Geometry: final body of the model. Coordinates: model frame, mm. A direction names the side the tool comes from. Give positions to 0.01 mm unless a question says otherwise; leave off trailing zeros. Order: outer loops, then holes, each group sorted by start corner. A loop starts at its lowest first (then second) coordinate and runs counter-clockwise, first axis right, second up. Notation, with made-up numbers: M -8,66.5 L 30,66.5 A32 ccw 30,101.5 Z; hole C -18.75,14.25 d9. An arc over 180 degrees is marked long. One line per item, written item: value. Start each with the question number.
```python
from build123d import *

# Parameters (mm, degrees)
F0_R     = 11
F1_DEPTH = 7


with BuildPart() as f1:
    # F0 (on Top) → F1 (new body)
    with BuildSketch(Plane.XY):
        with BuildLine():
            ThreePointArc((9.403824, 18.776797), (0, 21), (-9.403824, 18.776797))
            ThreePointArc((-9.403824, 18.776797), (-12.34349, 16.989357), (-14.951853, 14.745918))
            ThreePointArc((-14.951853, 14.745918), (-19.972187, 6.489357), (-20.763736, -3.141219))
            ThreePointArc((-20.763736, -3.141219), (-19.972187, -6.489357), (-18.644578, -9.663318))
            ThreePointArc((-18.644578, -9.663318), (-12.34349, -16.989357), (-3.42887, -20.718177))
            ThreePointArc((-3.42887, -20.718177), (0, -21), (3.42887, -20.718177))
            ThreePointArc((3.42887, -20.718177), (12.34349, -16.989357), (18.644578, -9.663318))
            ThreePointArc((18.644578, -9.663318), (19.972187, -6.489357), (20.763736, -3.141219))
            ThreePointArc((20.763736, -3.141219), (20.940851, -1.575046), (21, 0))
            ThreePointArc((21, 0), (19.429217, 7.969036), (14.951853, 14.745918))
            ThreePointArc((14.951853, 14.745918), (12.34349, 16.989357), (9.403824, 18.776797))
        make_face()
        Circle(F0_R, mode=Mode.SUBTRACT)
        with BuildLine():
            Line((-0.986697, 24.434563), (-0.986697, 39.987829))
            ThreePointArc((-0.986697, 39.987829), (-4.11855, 39.787404), (-7.225052, 39.342072))
            Line((-7.225052, 39.342072), (-9.403824, 18.776797))
            ThreePointArc((-9.403824, 18.776797), (0, 21), (9.403824, 18.776797))
            Line((9.403824, 18.776797), (7.225052, 39.342072))
            ThreePointArc((7.225052, 39.342072), (4.11855, 39.787404), (0.986697, 39.987829))
            Line((0.986697, 39.987829), (0.986697, 24.434563))
            Line((0.986697, 24.434563), (-0.986697, 24.434563))
        make_face()
        with BuildLine():
            Line((35.18387, 19.028802), (14.951853, 14.745918))
            ThreePointArc((14.951853, 14.745918), (19.429217, 7.969036), (21, 0))
            ThreePointArc((21, 0), (20.940851, -1.575046), (20.763736, -3.141219))
            Line((20.763736, -3.141219), (39.649198, 5.285936))
            ThreePointArc((39.649198, 5.285936), (39.112772, 8.37801), (38.335591, 11.418514))
            Line((38.335591, 11.418514), (23.543556, 6.612291))
            Line((23.543556, 6.612291), (22.933744, 8.4891))
            Line((22.933744, 8.4891), (37.725779, 13.295323))
            ThreePointArc((37.725779, 13.295323), (36.567368, 16.211958), (35.18387, 19.028802))
        make_face()
        with BuildLine():
            Line((28.96988, -27.581626), (18.644578, -9.663318))
            ThreePointArc((18.644578, -9.663318), (12.34349, -16.989357), (3.42887, -20.718177))
            Line((3.42887, -20.718177), (17.2795, -36.075184))
            ThreePointArc((17.2795, -36.075184), (20.054472, -34.609509), (22.706001, -32.930799))
            Line((22.706001, -32.930799), (13.564021, -20.347942))
            Line((13.564021, -20.347942), (15.16053, -19.188011))
            Line((15.16053, -19.188011), (24.30251, -31.770867))
            ThreePointArc((24.30251, -31.770867), (26.718427, -29.767863), (28.96988, -27.581626))
        make_face()
        with BuildLine():
            ThreePointArc((-3.42887, -20.718177), (-12.34349, -16.989357), (-18.644578, -9.663318))
            Line((-18.644578, -9.663318), (-28.96988, -27.581626))
            ThreePointArc((-28.96988, -27.581626), (-26.718427, -29.767863), (-24.30251, -31.770867))
            Line((-24.30251, -31.770867), (-15.16053, -19.188011))
            Line((-15.16053, -19.188011), (-13.564021, -20.347942))
            Line((-13.564021, -20.347942), (-22.706001, -32.930799))
            ThreePointArc((-22.706001, -32.930799), (-20.054472, -34.609509), (-17.2795, -36.075184))
            Line((-17.2795, -36.075184), (-3.42887, -20.718177))
        make_face()
        with BuildLine():
            ThreePointArc((-20.763736, -3.141219), (-19.972187, 6.489357), (-14.951853, 14.745918))
            Line((-14.951853, 14.745918), (-35.18387, 19.028802))
            ThreePointArc((-35.18387, 19.028802), (-36.567368, 16.211958), (-37.725779, 13.295323))
            Line((-37.725779, 13.295323), (-22.933744, 8.4891))
            Line((-22.933744, 8.4891), (-23.543556, 6.612291))
            Line((-23.543556, 6.612291), (-38.335591, 11.418514))
            ThreePointArc((-38.335591, 11.418514), (-39.112772, 8.37801), (-39.649198, 5.285936))
            Line((-39.649198, 5.285936), (-20.763736, -3.141219))
        make_face()
    extrude(amount=F1_DEPTH)


solid = f1.part
```
Q1. Section query B-B on y = 0. Return loops of the section in (x, z), and give its area (3 significant figures).
Q2. Mould query, pull axis Y, two halves, no side actions, for faces 1 (the face through (6, 11, 0)), 2 (the face through (-30.34, 1.13, 3.45)), 3 (the face through (-4.075, 39.792, 3.451)). Classes: +Y half, -Y half, draft (parallel to the pull), parting line (faces both ways), or undercut.
Q3. Section query C-C on x = 26.5. Return loops of the section in (y, z), and give its area (3 significant figures).
Q4. Contact query for flat-ended pins moving along their axis: pin 1 (4 mm diameter, centred on y = -18.5, z = 1, fed in from +X); pin 2 (0.6 mm diameter, centred on x = 0, z = 5, fed in from +Y); pin 3 (1 mm diameter, centred on x = 2.5, z = 3, fed in from +Y). Output: stop coordinate, or through.
Q5. Section query A-A on x = 0. Return loops of the section in (y, z), and give its area (3 significant figures).
Q6. Set-up query: faces 4 (the face through (-30.433, 10.926, 3.451)), 5 (the face through (25.209, 16.917, 3.451)), 6 (the face through (10.26, -28.29, 3.45)). Return all of +Z, -Z, +X, -X, +Y, -Y with unobstructed straight access to the full face (end or side cutting, diameter ignored); none if empty.
Q7. Section query D-D on y = -24. Return loops of the section in (x, z), and give its area (3 significant figures).
Q8. Ray query, line 1 along Y through (x, z) = (0, 3.75); line 2 along X through (y, z) = (-20, 2); line 3 along Y through (x, z) = (-24, 6). Return the intervals inside material, ascending. Write a range as [from, to].
Results below:
1. outline: M -27.8,0 L -11,0 L -11,7 L -27.8,7 Z; M 11,0 L 27.8,0 L 27.8,7 L 11,7 Z
1. area: 235 mm2
2. face 1: draft
2. face 2: undercut
2. face 3: +Y half
3. outline: M -29.96,0 L -23.3,0 L -23.3,7 L -29.96,7 Z; M -0.58,0 L 7.57,0 L 7.57,7 L -0.58,7 Z; M 9.65,0 L 17.19,0 L 17.19,7 L 9.65,7 Z
3. area: 157 mm2
4. pin 1: x = 24.89
4. pin 2: y = 24.43
4. pin 3: y = 39.95
5. outline: M -21,0 L -11,0 L -11,7 L -21,7 Z; M 11,0 L 24.43,0 L 24.43,7 L 11,7 Z
5. area: 164 mm2
6. face 4: +Z, -Z
6. face 5: +Z, -Z, +Y
6. face 6: +Z, -Z, -Y
7. outline: M -26.91,0 L -18.66,0 L -18.66,7 L -26.91,7 Z; M -16.22,0 L -6.39,0 L -6.39,7 L -16.22,7 Z; M 6.39,0 L 16.22,0 L 16.22,7 L 6.39,7 Z; M 18.66,0 L 26.91,0 L 26.91,7 L 18.66,7 Z
7. area: 253 mm2
8. line 1: [-21, -11], [11, 24.43]
8. line 2: [-24.6, -15.75], [-14.04, 14.04], [15.75, 24.6]
8. line 3: [-31.35, -18.96], [-1.7, 6.76], [8.84, 16.66]
